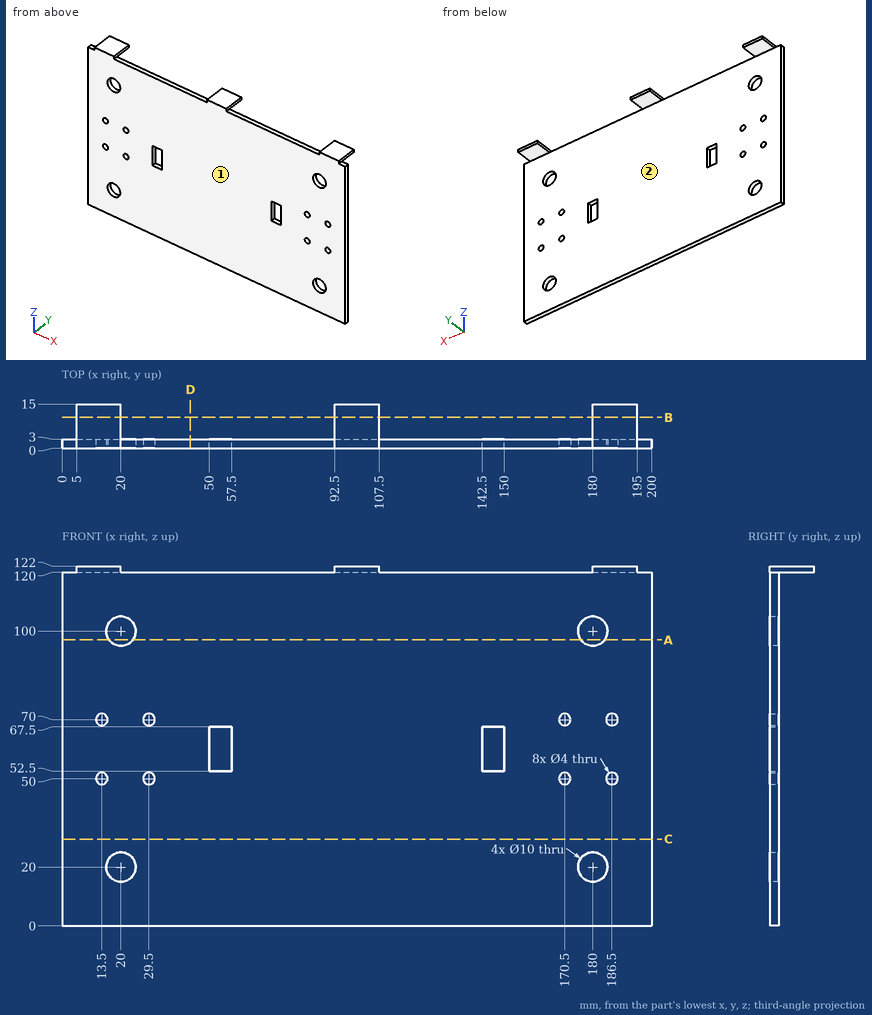
Could you check a few things on this drawing? It's one solid part, dimensions in mm from its lowest x, y, z. A direction names the side the tool comes from. Give positions to 0.01 mm unless a question says otherwise; leave off trailing zeros. Order: outer loops, then holes, each group sorted by start corner. A loop starts at its lowest first (then second) coordinate and runs counter-clockwise, first axis right, second up. Notation, with made-up numbers: (1.25, 71.5) - (5.25, 71.5) arc R20 ccw to (5.25, 94.5) - close; hole circle Ø3 at (72, 59.5). An arc over 180 degrees is marked (long way). One line per question, with ' | ' between items. Start each with the question number.
Item 1: I want a section at D-D on x = 43.5. Write out the boundary of the cut face in (y, z), then the cut area to 3 significant figures.
Item 2: I'm going to push flat-ended pins straight in: pin 1 Ø0.6 at (y, z) = (9, 121) entering from +X; pin 2 Ø6.5 at (x, z) = (186.5, 50) entering from +Y; pin 3 Ø13 at (x, z) = (20, 20) entering from -Y; pin 4 Ø2.5 at (x, y) = (1.5, 1) entering from +Z. Where does each tip first touch, or does it pass through?
Item 3: I want a section at B-B on y = 10.5. Write out the boundary of the cut face in (x, z), then the cut area to 3 significant figures.
Item 4: For the marked faces 1 and 2, which set-ups out of +Z, -Z, +X, -X, +Y, -Y let a thin tool reach every point of the face, with its end or its side?
Item 5: I want a section at C-C on z = 29.5. Write out the boundary of the cut face in (x, y).
Item 6: I need wall thicknesses on probe 1 along X at (y, z) = (1.3, 100); probe 2 along X at (y, z) = (0.95, 70); probe 3 along Z at (x, y) = (170.5, 2.35). Which ranges of each line are inside material? Lowest first, please. Write a range as [from, to].
Item 7: I want a section at A-A on z = 97. Write out the boundary of the cut face in (x, y).
Verdict:
1) outline: (0, 0) - (3, 0) - (3, 120) - (0, 120) - close | area: 360 mm^2
2) pin 1: x = 195 | pin 2: y = 3 | pin 3: y = 0 | pin 4: z = 120
3) outline: (5, 120) - (20, 120) - (20, 122) - (5, 122) - close; (92.5, 120) - (107.5, 120) - (107.5, 122) - (92.5, 122) - close; (180, 120) - (195, 120) - (195, 122) - (180, 122) - close | area: 90.0 mm^2
4) face 1: +Z, -Z, +X, -X, -Y | face 2: -Z, +X, -X, +Y
5) outline: (0, 0) - (200, 0) - (200, 3) - (0, 3) - close
6) probe 1: [0, 15], [25, 175], [185, 200] | probe 2: [0, 11.5], [15.5, 27.5], [31.5, 168.5], [172.5, 184.5], [188.5, 200] | probe 3: [0, 48], [52, 68], [72, 120]
7) outline: (0, 0) - (16, 0) - (16, 3) - (0, 3) - close; (24, 0) - (176, 0) - (176, 3) - (24, 3) - close; (184, 0) - (200, 0) - (200, 3) - (184, 3) - close
